from build123d import *

# Parameters (mm, degrees)
SKETCH054_W     = 35
SKETCH054_H     = 70
PAD009_DEPTH    = 7
SKETCH055_R     = 1.6
SKETCH055_R_2   = 2.4
POCKET035_DEPTH = 10
SKETCH056_R     = 3.25
POCKET036_DEPTH = 2.5
FILLET004_R     = 5


with BuildPart() as part:
    # Sketch054 → Pad009 (new body)
    with BuildSketch(Plane.XY):
        Rectangle(SKETCH054_W, SKETCH054_H)
    extrude(amount=PAD009_DEPTH)

    # Sketch055 (on Face6 of Pad009) → Pocket035 (cut)
    with BuildSketch(Plane.XY.offset(7)):
        with Locations((7.5, 25)):
            Circle(SKETCH055_R)
        with Locations((-9.25, 0)):
            Circle(SKETCH055_R)
        with Locations((7.5, -25)):
            Circle(SKETCH055_R)
        with Locations((-8.8388347648, 8.8388347648)):
            Circle(SKETCH055_R_2)
        with Locations((8.8388347648, 8.8388347648)):
            Circle(SKETCH055_R_2)
        with Locations((-8.8388347648, -8.8388347648)):
            Circle(SKETCH055_R_2)
        with Locations((8.8388347648, -8.8388347648)):
            Circle(SKETCH055_R_2)
    extrude(amount=-POCKET035_DEPTH, mode=Mode.SUBTRACT)

    # Sketch056 (on Face5 of Pocket035) → Pocket036 (cut)
    with BuildSketch(Plane.XY.offset(7)):
        with Locations((-9.25, 0)):
            Circle(SKETCH056_R)
        with Locations((7.5, 25)):
            Circle(SKETCH056_R)
        with Locations((7.5, -25)):
            Circle(SKETCH056_R)
    extrude(amount=-POCKET036_DEPTH, mode=Mode.SUBTRACT)

    # Fillet004
    fillet004_edges = [part.edges().sort_by_distance(p)[0] for p in [
        (-17.5, -35, 3.5),
        (17.5, -35, 3.5),
        (-17.5, 35, 3.5),
        (17.5, 35, 3.5),
    ]]
    fillet(fillet004_edges, radius=FILLET004_R)


solid = part.part
Geometry check sheet. Reference: the model listing, model coordinates, mm. A direction names the side the tool comes from. Give positions to 0.01 mm unless a question says otherwise; leave off trailing zeros. Loops run counter-clockwise (first coordinate to the right, second up) from the corner with the lowest first, then second, coordinate; pieces in that order, holes last. Notation, with made-up numbers: (-28, 43) -> (29, 43) arc R24 cw to (29, 70) -> close; hole circle Ø5 at (59.5, -2.5). An arc over 180 degrees is marked (long way). Answer in a Markdown table with one row per item. Add a question column.
1) Cross-section at D-D on x = 7.5. Record the boundary of the cut face in (y, z), and give its area (3 significant figures).
2) Set-up check for faces 1 (the face through (6.23, 24.03, 2.28)), 2 (the face through (4.921, -26.978, 5.768)): record each of +Z, -Z, +X, -X, +Y, -Y from which the full face is reachable in a straight line by a thin tool's end or side.
3) Gauge pin test, flat ends, axial feed: P1, Ø6, axis at x = -8.84, y = 8.84, coming from the -Z side; P2, Ø2, axis at x = 8, y = -24.5, coming from the +Z side. Record the tip position at first contact, or that the pin passes through.
4) Material ranges on probe 1 along Y at (x, z) = (10.5, 1); probe 2 along Y at (x, z) = (-7, 2); probe 3 along X at (y, z) = (-7, 2), recorded low to high. Write a range as from..to.
5) Draft check along Y on faces 3 (the face through (-16.07, -33.5, 3.55)), 4 (the face through (10.129, -6.815, 3.549)), 5 (the face through (16, 33.57, 3.55)), 6 (the face through (6, -26, 4.5)). Enter one of: pulls with the +Y half, pulls with the -Y half, needs draft (parallel to the pull), parting line crosses it, or undercut.
6) Cross-section at A-A on y = 25. Record the boundary of the cut face in (x, z).
7) Cross-section at B-B on x = -9.25. Record the boundary of the cut face in (y, z).
8) Cross-section at C-C on z = 1.5. Record the boundary of the cut face in (x, y).
Outcome:
| question | item | result |
|---|---|---|
| 1 | outline | (-35, 0) -> (-26.6, 0) -> (-26.6, 4.5) -> (-28.25, 4.5) -> (-28.25, 7) -> (-35, 7) -> close; (-23.4, 0) -> (-10.83, 0) -> (-10.83, 7) -> (-21.75, 7) -> (-21.75, 4.5) -> (-23.4, 4.5) -> close; (-6.85, 0) -> (6.85, 0) -> (6.85, 7) -> (-6.85, 7) -> close; (10.83, 0) -> (23.4, 0) -> (23.4, 4.5) -> (21.75, 4.5) -> (21.75, 7) -> (10.83, 7) -> close; (26.6, 0) -> (35, 0) -> (35, 7) -> (28.25, 7) -> (28.25, 4.5) -> (26.6, 4.5) -> close |
| 1 | area | 373 mm^2 |
| 2 | face 1 | +Z, -Z |
| 2 | face 2 | +Z |
| 3 | P1 | stops at z = 0 |
| 3 | P2 | stops at z = 4.5 |
| 4 | probe 1 | y = -35..-10.57, -7.11..7.11, 10.57..35 |
| 4 | probe 2 | y = -35..-10.38, -7.3..7.3, 10.38..35 |
| 4 | probe 3 | x = -17.5..-10.38, -7.3..7.3, 10.38..17.5 |
| 5 | face 3 | pulls with the -Y half |
| 5 | face 4 | undercut |
| 5 | face 5 | pulls with the +Y half |
| 5 | face 6 | undercut |
| 6 | outline | (-17.5, 0) -> (5.9, 0) -> (5.9, 4.5) -> (4.25, 4.5) -> (4.25, 7) -> (-17.5, 7) -> close; (9.1, 0) -> (17.5, 0) -> (17.5, 7) -> (10.75, 7) -> (10.75, 4.5) -> (9.1, 4.5) -> close |
| 7 | outline | (-35, 0) -> (-11.2, 0) -> (-11.2, 7) -> (-35, 7) -> close; (-6.47, 0) -> (-1.6, 0) -> (-1.6, 4.5) -> (-3.25, 4.5) -> (-3.25, 7) -> (-6.47, 7) -> close; (1.6, 0) -> (6.47, 0) -> (6.47, 7) -> (3.25, 7) -> (3.25, 4.5) -> (1.6, 4.5) -> close; (11.2, 0) -> (35, 0) -> (35, 7) -> (11.2, 7) -> close |
| 8 | outline | (-17.5, -30) arc R5 ccw to (-12.5, -35) -> (12.5, -35) arc R5 ccw to (17.5, -30) -> (17.5, 30) arc R5 ccw to (12.5, 35) -> (-12.5, 35) arc R5 ccw to (-17.5, 30) -> close; hole circle Ø4.8 at (-8.84, -8.84); hole circle Ø4.8 at (-8.84, 8.84); hole circle Ø3.2 at (-9.25, 0); hole circle Ø3.2 at (7.5, -25); hole circle Ø3.2 at (7.5, 25); hole circle Ø4.8 at (8.84, -8.84); hole circle Ø4.8 at (8.84, 8.84) |
